Geometry check sheet. Reference: the model listing, model coordinates, mm. A direction names the side the tool comes from. Coordinates: 2 decimals unless noted, no trailing zeros. Order: outer loops, then holes, each group sorted by start corner. A loop starts at its lowest first (then second) coordinate and runs counter-clockwise, first axis right, second up. Notation, with made-up numbers: (74, 7.25) - (131, 7.25) arc R19 cw to (131, 33.25) - close; hole circle Ø8 at (47, 9.5). An arc over 180 degrees is marked (long way). Return JSON: item names as keys, results as strings. Group by question number.
Item 1: Scan lines: probe 1 along X at (y, z) = (-20, 25); probe 2 along Y at (x, z) = (65, 19); probe 3 along X at (y, z) = (-20, 19). Record each from-to range of solid material in increasing order.
Item 2: Section check C-C on y = -20. Enter the section's corners in (x, z).
Item 3: Gauge pin test, flat ends, axial feed: pin 1 (12 mm diameter, centred on x = 26.5, y = -31, fed in from +Z); pin 2 (6 mm diameter, centred on y = -12.5, z = 22, fed in from -X); pin 3 (7.5 mm diameter, centred on y = -17, z = 30.5, fed in from -X); pin 4 (13.5 mm diameter, centred on x = 65, y = -20, fed in from +Z). Record the tip position at first contact, or that the pin passes through.
Item 4: Tool access check on faces 4 (the flat face through (87, 0, 20)), 5 (the flat face through (43, -2, 27)), 6 (the flat face through (3.4, -3.1, 3.5)), 7 (the flat face through (40, -20, 28)), 8 (the flat face through (43, -38, 27)). Record the directions out of +Z, -Z, +X, -X, +Y, -Y that give a thin tool (end or side, any length) a straight path to the whole face; none if there is none.
Item 5: Draft check along Y on faces 1 (the cylindrical face through (61.074, -18.372, 20.28)), 2 (the flat face through (0, -20, 10)), 3 (the flat face through (43.4, -36.9, 36.5)). Enter one of: pulls with the +Y half, pulls with the -Y half, needs draft (parallel to the pull), parting line crosses it, or undercut.
Item 6: Section check A-A on z = 25.5. Enter the section's corners in (x, y).
Item 7: Section check D-D on x = 43.5. Enter the section's corners in (y, z).
Item 8: Section check B-B on x = 65. Enter the section's corners in (y, z).
from build123d import *

# Parameters (mm, degrees)
F1_DEPTH = 40
F2_SIZE  = 5
F4_D     = 8.5
F6_D     = 8.5
F7_SIZE  = 5
F8_SIZE  = 5


with BuildPart() as f1:
    # F0 (on Front) → F1 (new body)
    with BuildSketch(Plane.XZ):
        Polygon((0, 20), (0, 0), (140, 0), (140, 40), (40, 40), (40, 20), align=None)
    extrude(amount=F1_DEPTH)

    # F2
    f2_edges = [f1.edges().sort_by_distance(p)[0] for p in [
        (40, -20, 40),
        (40, -40, 30),
        (40, 0, 30),
        (0, -20, 20),
        (0, -40, 10),
        (0, -20, 0),
        (0, 0, 10),
        (90, -40, 40),
        (70, -40, 0),
        (90, 0, 40),
        (70, 0, 0),
    ]]
    chamfer(f2_edges, length=F2_SIZE)

    # F4 (through all)
    with Locations(Plane(origin=(0, 0, 0), x_dir=(1, 0, 0), z_dir=(0, 0, -1))):
        with Locations((115, 20)):
            Hole(F4_D / 2)

    # F6 (through all)
    with Locations(Plane(origin=(0, 0, 0), x_dir=(1, 0, 0), z_dir=(0, 0, -1))):
        with Locations((65, 20)):
            Hole(F6_D / 2)

    # F7
    f7_edges = [f1.edges().sort_by_distance(p)[0] for p in [
        (25, 0, 20),
    ]]
    chamfer(f7_edges, length=F7_SIZE)

    # F8
    f8_edges = [f1.edges().sort_by_distance(p)[0] for p in [
        (25, -40, 20),
    ]]
    chamfer(f8_edges, length=F8_SIZE)


solid = f1.part
Computed:
{
 "1": {"probe 1": "x = 40 to 60.75, 69.25 to 110.75, 119.25 to 140", "probe 2": "y = -40 to -24.25, -15.75 to 0", "probe 3": "x = 4 to 60.75, 69.25 to 110.75, 119.25 to 140"},
 "2": {"outline": "(0, 5) - (5, 0) - (60.75, 0) - (60.75, 40) - (45, 40) - (40, 35) - (40, 20) - (5, 20) - (0, 15) - close; (69.25, 0) - (110.75, 0) - (110.75, 40) - (69.25, 40) - close; (119.25, 0) - (140, 0) - (140, 40) - (119.25, 40) - close"},
 "3": {"pin 1": "stops at z = 20", "pin 2": "stops at x = 4", "pin 3": "stops at x = 40", "pin 4": "stops at z = 40"},
 "4": {"face 4": "+Z, -Z, +X, -X, +Y", "face 5": "+Z, -X, +Y", "face 6": "-Z, -X, +Y", "face 7": "+Z, -X, +Y, -Y", "face 8": "+Z, -X, -Y"},
 "5": {"face 1": "undercut", "face 2": "needs draft", "face 3": "pulls with the -Y half"},
 "6": {"outline": "(40, -35) - (45, -40) - (140, -40) - (140, 0) - (45, 0) - (40, -5) - close; hole circle Ø8.5 at (65, -20); hole circle Ø8.5 at (115, -20)"},
 "7": {"outline": "(-40, 5) - (-35, 0) - (-5, 0) - (0, 5) - (0, 15) - (-1.5, 16.5) - (-1.5, 35) - (-5, 38.5) - (-35, 38.5) - (-38.5, 35) - (-38.5, 16.5) - (-40, 15) - close"},
 "8": {"outline": "(-40, 5) - (-35, 0) - (-24.25, 0) - (-24.25, 40) - (-35, 40) - (-40, 35) - close; (-15.75, 0) - (-5, 0) - (0, 5) - (0, 35) - (-5, 40) - (-15.75, 40) - close"}
}
